The drawing under review shows one solid part. Ordinate dimensions are in mm from its lowest x, y, z. A direction names the side the tool comes from. Give positions to 0.01 mm unless a question says otherwise; leave off trailing zeros. Order: outer loops, then holes, each group sorted by start corner. A loop starts at its lowest first (then second) coordinate and runs counter-clockwise, first axis right, second up. Notation, with made-up numbers: (24, 77) -> (37, 77) arc R4 ccw to (37, 84) -> close; hole circle Ø5 at (24, -4). An arc over 180 degrees is marked (long way). One line per item, written item: value. Start each with the question number.
1) Tool access review of the marked faces 1 and 2: name each direction out of +Z, -Z, +X, -X, +Y, -Y from which nothing blocks a thin tool from reaching the whole face with its end or side.
2) The part is to be moulded in two halves that separate along Z. For the marked faces 3, 4 and 5, say which applies: released by +Z, released by -Z, zero draft, split by the parting line, or undercut.
3) Wall thickness on line 1 along Z through (x, y) = (25, 36.5); line 2 along Y through (x, z) = (18.5, 17.25); line 3 along X through (y, z) = (27, 7.25): over which ranges is each line inside the solid? List them lowest first. Write a range as from..to.
4) For pin 1 (10 mm diameter, centred on x = 11.5, z = 9.5, fed in from +Y); pin 2 (5 mm diameter, centred on x = 28, z = 14, fed in from +Y); pin 3 (4 mm diameter, centred on y = 12, z = 15, fed in from -X), all flat-tipped, find the tip position at first contact; note any pin that passes through.
5) Consider section A-A (y = 19.9). State the section outline as (x, z) points.
6) Consider section C-C (z = 13.75). State the section outline as (x, y) points, plus the area to 3 significant figures.
7) Consider section D-D (z = 21.75). State the section outline as (x, y) points (3 decimals).
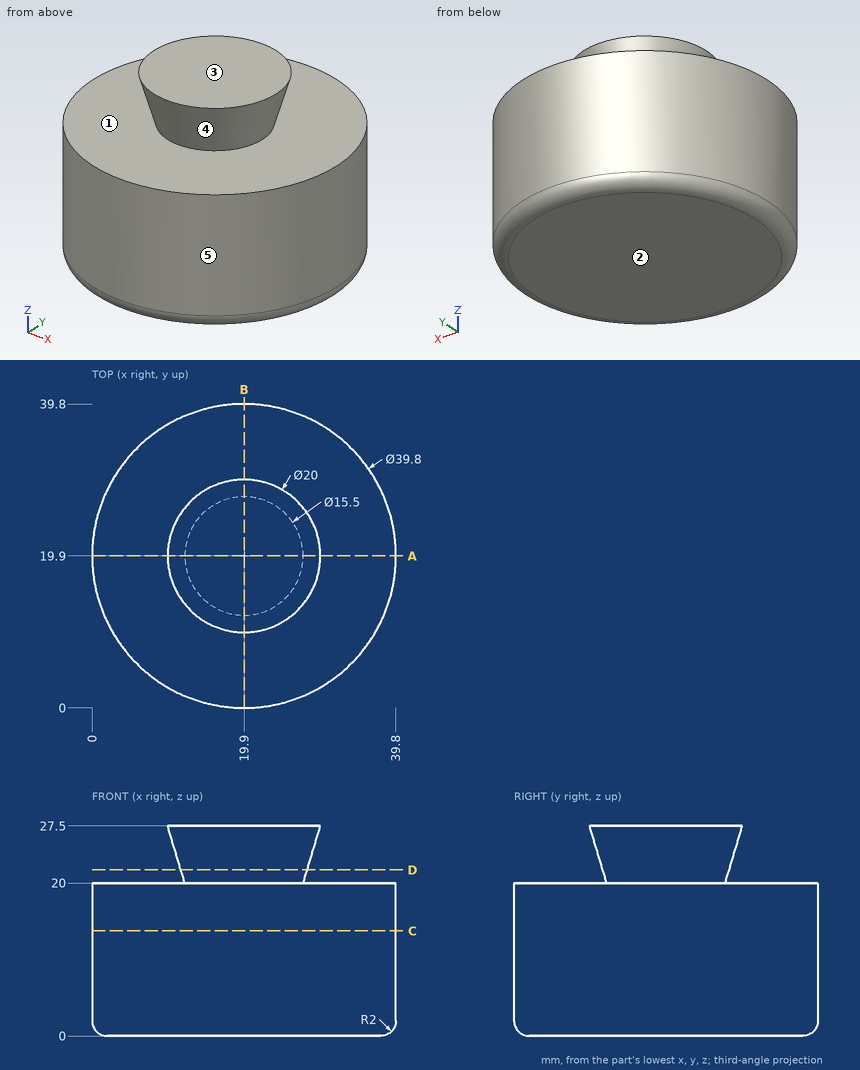
Checked values:
1. face 1: none
1. face 2: -Z, +X, -X, +Y, -Y
2. face 3: released by +Z
2. face 4: undercut
2. face 5: zero draft
3. line 1: z = 0..20
3. line 2: y = 0.05..39.75
3. line 3: x = 1.31..38.49
4. pin 1: stops at y = 39.51
4. pin 2: stops at y = 39
4. pin 3: stops at x = 0.89
5. outline: (0, 2) arc R2 ccw to (2, 0) -> (37.8, 0) arc R2 ccw to (39.8, 2) -> (39.8, 20) -> (27.65, 20) -> (29.9, 27.5) -> (9.9, 27.5) -> (12.15, 20) -> (0, 20) -> close
6. outline: circle Ø39.8 at (19.9, 19.9)
6. area: 1,240 mm^2
7. outline: circle Ø16.55 at (19.9, 19.9)
